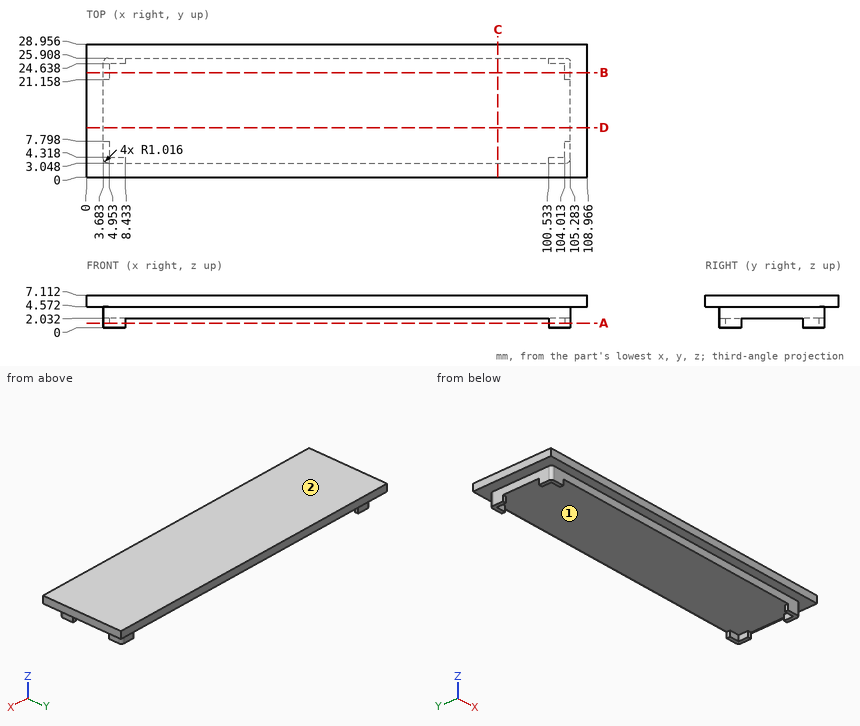
Print and shaded views of the part. All mm, measured from the part's lowest x, y and z. Give positions to 0.01 mm unless a question says otherwise; leave off trailing zeros. Order: outer loops, then holes, each group sorted by start corner. A loop starts at its lowest first (then second) coordinate and runs counter-clockwise, first axis right, second up. Notation, with made-up numbers: (78.5, 57.5) - (116.5, 57.5) arc R14 cw to (116.5, 71.5) - close; hole circle Ø9 at (13.25, 6). An arc over 180 degrees is marked (long way). Use a Markdown table: item, result.
1) Flat gauge pins, fed straight in: P1, Ø0.6, axis at x = 6, z = 0.5, coming from the -Y side; P2, Ø2, axis at y = 7, z = 1, coming from the +X side; P3, Ø1, axis at x = 50.5, y = 6.5, coming from the -Z side; P4, Ø2, axis at y = 19, z = 5, coming from the -X side. Where does each tip first touch, or does it go through?
Checked values:
| item | result |
|---|---|
| P1 | y = 3.05 |
| P2 | x = 105.28 |
| P3 | z = 2.03 |
| P4 | x = 0 |
2) Probe L1, parallel to X at y = 6.5, z = 1.25; L2, parallel to Y at x = 81, z = 3; L3, parallel to Z at x = 81, y = 17.5. List the from-to ranges inside material, lowest first. Write a range as from..to.
Checked values:
| item | result |
|---|---|
| L1 | 3.68..4.95, 104.01..105.28 |
| L2 | 3.05..25.91 |
| L3 | 2.03..7.11 |
3) Saw through at B-B on y = 22.75. List the corners of the cut face in (x, z).
Checked values:
| item | result |
|---|---|
| outline | (0, 4.57) - (3.68, 4.57) - (3.68, 0) - (4.95, 0) - (4.95, 2.03) - (104.01, 2.03) - (104.01, 0) - (105.28, 0) - (105.28, 4.57) - (108.97, 4.57) - (108.97, 7.11) - (0, 7.11) - close |
4) Two-plate mould, pull along X, no slides. Class the marked faces 1 and 2: +X half, -X half, draft (parallel to the pull), parting line (faces both ways), or undercut.
Checked values:
| item | result |
|---|---|
| face 1 | undercut |
| face 2 | draft |
5) Saw through at C-C on x = 89.5. List the corners of the cut face in (y, z).
Checked values:
| item | result |
|---|---|
| outline | (0, 4.57) - (3.05, 4.57) - (3.05, 2.03) - (25.91, 2.03) - (25.91, 4.57) - (28.96, 4.57) - (28.96, 7.11) - (0, 7.11) - close |
6) Saw through at D-D on y = 10.75. List the corners of the cut face in (x, z), plus the area to 3 significant figures.
Checked values:
| item | result |
|---|---|
| outline | (0, 4.57) - (3.68, 4.57) - (3.68, 2.03) - (105.28, 2.03) - (105.28, 4.57) - (108.97, 4.57) - (108.97, 7.11) - (0, 7.11) - close |
| area | 535 mm² |
7) Saw through at A-A on z = 1. List the corners of the cut face in (x, y).
Checked values:
| item | result |
|---|---|
| outline | (3.68, 4.06) arc R1.02 ccw to (4.7, 3.05) - (8.43, 3.05) - (8.43, 4.32) - (4.95, 4.32) - (4.95, 7.8) - (3.68, 7.8) - close; (3.68, 21.16) - (4.95, 21.16) - (4.95, 24.64) - (8.43, 24.64) - (8.43, 25.91) - (4.7, 25.91) arc R1.02 ccw to (3.68, 24.89) - close; (100.53, 3.05) - (104.27, 3.05) arc R1.02 ccw to (105.28, 4.06) - (105.28, 7.8) - (104.01, 7.8) - (104.01, 4.32) - (100.53, 4.32) - close; (100.53, 24.64) - (104.01, 24.64) - (104.01, 21.16) - (105.28, 21.16) - (105.28, 24.89) arc R1.02 ccw to (104.27, 25.91) - (100.53, 25.91) - close |
